Check sheet for the modelled part. Datum: model origin and axes. Units: mm. A direction names the side the tool comes from. Round coordinates to 2 decimals unless told otherwise and drop trailing zeros. Loops run counter-clockwise (first coordinate to the right, second up) from the corner with the lowest first, then second, coordinate; pieces in that order, holes last. Notation, with made-up numbers: (30.5, 79.25) - (38.5, 79.25) arc R32 ccw to (38.5, 110.25) - close; hole circle Ø2 at (-15, 8.25). An arc over 180 degrees is marked (long way). Return JSON: item names as keys, results as strings.
from build123d import *

# Parameters (mm, degrees)
SKETCH1_R          = 2.4892
BASE_FLANGE1_DEPTH = 3.175
FILLET2_R          = 4.7625


# Sheet-metal steps are written as plain solids
with BuildPart() as part:
    # Sketch1 → Base-Flange1 (new body)
    with BuildSketch(Plane.XY):
        Polygon((-15.24, 31.75), (-34.925, 31.75), (-34.925, -31.75), (34.925, -31.75), (34.925, -7.62), (-15.24, -7.62), align=None)
        with Locations((-25.4, -6.35)):
            Circle(SKETCH1_R, mode=Mode.SUBTRACT)
        with Locations((-25.4, 6.35)):
            Circle(SKETCH1_R, mode=Mode.SUBTRACT)
        with Locations((-1.5875, -19.05)):
            Circle(SKETCH1_R, mode=Mode.SUBTRACT)
        with Locations((15.875, -19.05)):
            Circle(SKETCH1_R, mode=Mode.SUBTRACT)
        with Locations((28.575, -19.05)):
            Circle(SKETCH1_R, mode=Mode.SUBTRACT)
    extrude(amount=-BASE_FLANGE1_DEPTH)

    # Fillet2
    fillet2_edges = [part.edges().sort_by_distance(p)[0] for p in [
        (-34.925, -31.75, -1.5875),
        (34.925, -31.75, -1.5875),
        (34.925, -7.62, -1.5875),
        (-15.24, -7.62, -1.5875),
        (-15.24, 31.75, -1.5875),
        (-34.925, 31.75, -1.5875),
    ]]
    fillet(fillet2_edges, radius=FILLET2_R)


solid = part.part
Q1. Scan lines: probe 1 along Y at (x, z) = (-25.4, -0.65); probe 2 along X at (y, z) = (-19.5, -1.35) (3 decimals); probe 3 along X at (y, z) = (3, -0.7) (3 decimals). Record each from-to range of solid material in increasing order. Write a range as [from, to].
Answer key:
{"probe 1": "y = [-31.75, -8.84], [-3.86, 3.86], [8.84, 31.75]", "probe 2": "x = [-34.925, -4.036], [0.861, 13.427], [18.323, 26.127], [31.023, 34.925]", "probe 3": "x = [-34.925, -15.24]"}
Q2. Tool access check on faces 1 (the face through (-15.24, 12, -2)), 2 (the face through (33.493, -30.392, -1.61)). Record the directions out of +Z, -Z, +X, -X, +Y, -Y that give a thin tool (end or side, any length) a straight path to the whole face; none if there is none.
Answer key:
{"face 1": "+Z, -Z, +X, +Y", "face 2": "+Z, -Z, +X, -Y"}
Q3. Sectioned sample at B-B (z = -0.75). State how many separate pieces and enclosed holes the cut face has, plus the area to 3 significant figures.
Answer key:
{"separate pieces": "1", "enclosed holes": "5", "area": "2,340 mm²"}
Q4. Sectioned sample at C-C (y = 6.35). Enter the section's corners in (x, z) (3 decimals).
Answer key:
{"outline": "(-34.925, -3.175) - (-27.889, -3.175) - (-27.889, 0) - (-34.925, 0) - close; (-22.911, -3.175) - (-15.24, -3.175) - (-15.24, 0) - (-22.911, 0) - close"}
Q5. Draft check along Y on faces 3 (the face through (-1.91, -16.58, -1.57)), 4 (the face through (0, -31.75, -2)), 5 (the face through (-16.67, 30.39, -1.61)), 6 (the face through (34.925, -20, -2)). Enter one of: released by +Y, released by -Y, zero draft, split by the parting line, or undercut.
Answer key:
{"face 3": "undercut", "face 4": "released by -Y", "face 5": "released by +Y", "face 6": "zero draft"}
Q6. Sectioned sample at D-D (y = -19.05). Enter the section's corners in (x, z) (3 decimals).
Answer key:
{"outline": "(-34.925, -3.175) - (-4.077, -3.175) - (-4.077, 0) - (-34.925, 0) - close; (0.902, -3.175) - (13.386, -3.175) - (13.386, 0) - (0.902, 0) - close; (18.364, -3.175) - (26.086, -3.175) - (26.086, 0) - (18.364, 0) - close; (31.064, -3.175) - (34.925, -3.175) - (34.925, 0) - (31.064, 0) - close"}
Q7. Depth check by flat-ended pin: P1, Ø1.6, axis at y = 7.5, z = -2.5, coming from the +X side; P2, Ø4, axis at x = -25.4, y = -6.35, coming from the +Z side (3 decimals); P3, Ø1.6, axis at x = 10, z = -1.5, coming from the +Y side. Enter the tip coordinate at first touch or a pass-through.
Answer key:
{"P1": "stops at x = -15.24", "P2": "passes through", "P3": "stops at y = -7.62"}
Q8. Sectioned sample at A-A (x = -25.4). Enter the section's corners in (y, z) (3 decimals).
Answer key:
{"outline": "(-31.75, -3.175) - (-8.839, -3.175) - (-8.839, 0) - (-31.75, 0) - close; (-3.861, -3.175) - (3.861, -3.175) - (3.861, 0) - (-3.861, 0) - close; (8.839, -3.175) - (31.75, -3.175) - (31.75, 0) - (8.839, 0) - close"}
